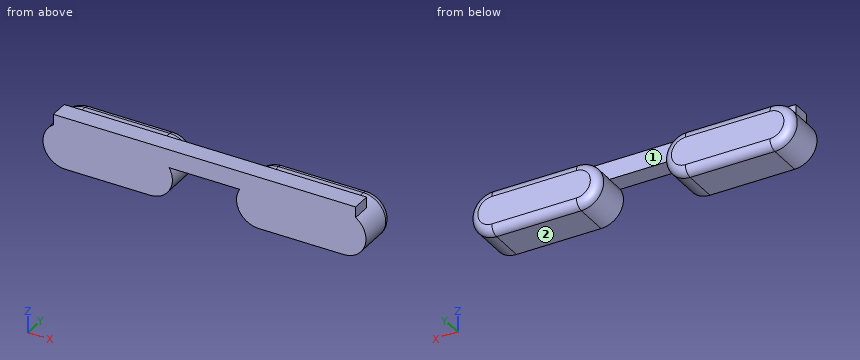
from build123d import *

# Parameters (mm, degrees)
SKETCH007_W  = 25
SKETCH007_H  = 1.5
PAD001_DEPTH = 1.55
PAD002_DEPTH = 3.5
FILLET002_R  = 0.7


with BuildPart() as part:
    # Sketch007 → Pad001 (new body)
    with BuildSketch(Plane.XZ):
        with Locations((0, 0.1)):
            Rectangle(SKETCH007_W, SKETCH007_H)
    extrude(amount=-PAD001_DEPTH)

    # Sketch008 → Pad002 (join)
    with BuildSketch(Plane.XZ):
        with BuildLine():
            ThreePointArc((-11.5, 0.25), (-13.35, -1.6), (-11.5, -3.45))
            Line((-11.5, -3.45), (-4.5, -3.45))
            ThreePointArc((-4.5, -3.45), (-2.65, -1.6), (-4.5, 0.25))
            Line((-4.5, 0.25), (-11.5, 0.25))
        make_face()
    pad002 = extrude(amount=-PAD002_DEPTH)

    # Mirrored001: Pad002 across Sketch008 V_Axis
    add(pad002.mirror(Plane(origin=(0, 0, 0), x_dir=(0, -1, 0), z_dir=(1, 0, 0))))

    # Fillet002
    fillet002_edges = [part.edges().sort_by_distance(p)[0] for p in [
        (13.35, 3.5, -1.6),
        (8, 3.5, -3.45),
        (2.65, 3.5, -1.6),
        (8, 3.5, 0.25),
        (-13.35, 3.5, -1.6),
        (-8, 3.5, -3.45),
        (-2.65, 3.5, -1.6),
        (-8, 3.5, 0.25),
    ]]
    fillet(fillet002_edges, radius=FILLET002_R)


solid = part.part
Model file for the job. Use its own axes, mm. Face numbers are marked on the shaded views. A direction names the side the tool comes from. Coordinates: 2 decimals unless noted, no trailing zeros. Order: outer loops, then holes, each group sorted by start corner. A loop starts at its lowest first (then second) coordinate and runs counter-clockwise, first axis right, second up. Notation, with made-up numbers: (67.25, 27) -> (109.25, 27) arc R21 ccw to (109.25, 47) -> close; hole circle Ø3 at (52, -7.75). An arc over 180 degrees is marked (long way). Return JSON: item names as keys, results as strings. Group by question number.
Item 1: Saw through at D-D on x = 6.75. Write the cut outline in (y, z).
Item 2: Flat gauge pins, fed straight in: P1, Ø0.8, axis at x = 0.5, y = 0.5, coming from the -Z side; P2, Ø1.2, axis at x = -1, z = 0.5, coming from the +Y side. Where does each tip first touch, or does it go through?
Item 3: Wall check: line 1 along Z through (x, y) = (7.75, 2.8); line 2 along Z through (x, y) = (-2.5, 0.9); line 3 along Y through (x, z) = (5.75, 0.6). Give the ranges that are in metal, low to high. Write a range as [from, to].
Item 4: Saw through at C-C on y = 0.9. Write the cut outline in (x, z), then the cut area to 3 significant figures.
Item 5: Saw through at A-A on z = -1.6. Write the cut outline in (x, y).
Item 6: Tool access for the marked faces 1 and 2: list every direction of +Z, -Z, +X, -X, +Y, -Y with a clear straight run to the whole face (end or side of a thin tool).
Item 7: Saw through at B-B on y = 2.3. Write the cut outline in (x, z).
Values found:
{
 "1": {"outline": "(0, -3.45) -> (2.8, -3.45) arc R0.7 ccw to (3.5, -2.75) -> (3.5, -0.45) arc R0.7 ccw to (2.8, 0.25) -> (1.55, 0.25) -> (1.55, 0.85) -> (0, 0.85) -> close"},
 "2": {"P1": "stops at z = -0.65", "P2": "stops at y = 1.55"},
 "3": {"line 1": "z = [-3.45, 0.25]", "line 2": "z = [-0.65, 0.85]", "line 3": "y = [0, 1.55]"},
 "4": {"outline": "(-12.5, -0.04) arc R1.85 ccw to (-11.5, -3.45) -> (-4.5, -3.45) arc R1.85 ccw to (-2.91, -0.65) -> (2.91, -0.65) arc R1.85 ccw to (4.5, -3.45) -> (11.5, -3.45) arc R1.85 ccw to (12.5, -0.04) -> (12.5, 0.85) -> (-12.5, 0.85) -> close", "area": "94.6 mm2"},
 "5": {"outline": "(-13.35, 0) -> (-2.65, 0) -> (-2.65, 2.8) arc R0.7 ccw to (-3.35, 3.5) -> (-12.65, 3.5) arc R0.7 ccw to (-13.35, 2.8) -> close; (2.65, 0) -> (13.35, 0) -> (13.35, 2.8) arc R0.7 ccw to (12.65, 3.5) -> (3.35, 3.5) arc R0.7 ccw to (2.65, 2.8) -> close"},
 "6": {"face 1": "+Z, +Y", "face 2": "-Z, +X, -X, +Y, -Y"},
 "7": {"outline": "(-11.5, -3.45) -> (-4.5, -3.45) arc R1.85 ccw to (-4.5, 0.25) -> (-11.5, 0.25) arc R1.85 ccw to start; (4.5, -3.45) -> (11.5, -3.45) arc R1.85 ccw to (11.5, 0.25) -> (4.5, 0.25) arc R1.85 ccw to start"}
}
